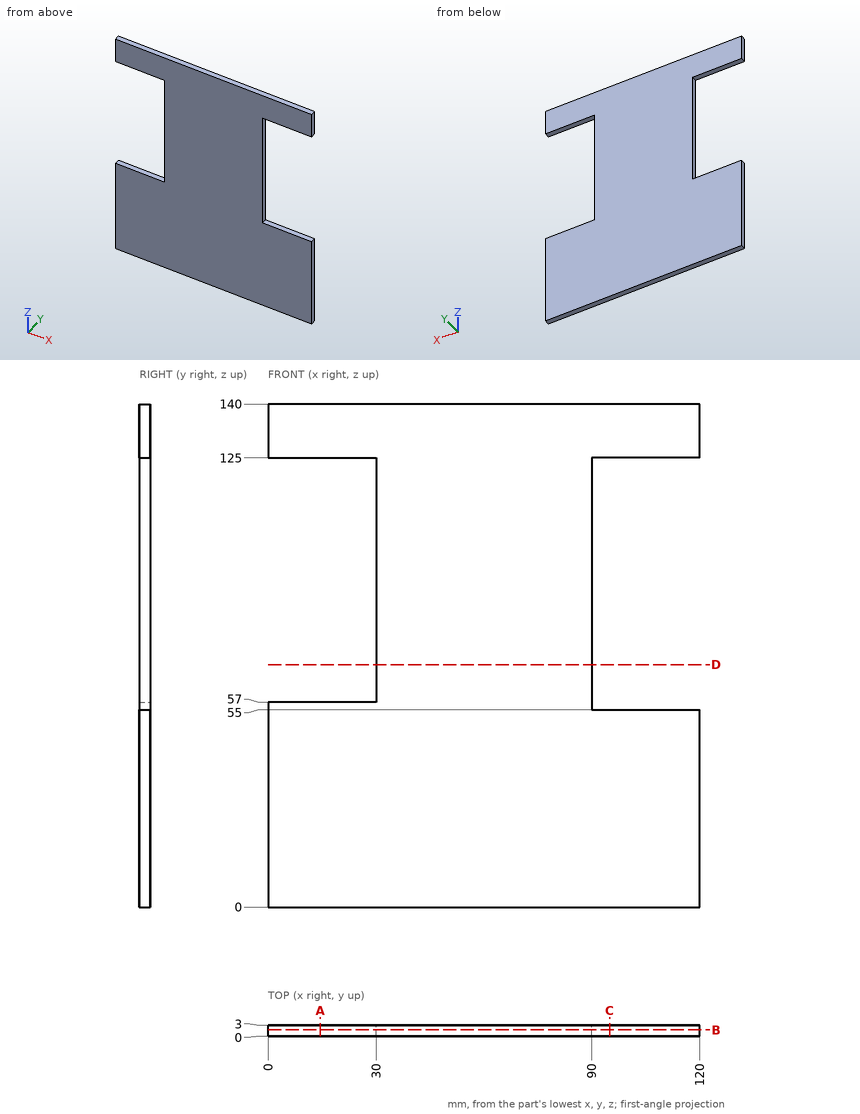
Source: three-view drawing plus pictorial views. Frame: mm from the lowest corner of the part. Coordinates: 2 decimals unless noted, no trailing zeros. Write each loop counter-clockwise with the first axis right and the second up, starting at its lowest first coordinate (ties: lowest second). Pieces come first, ordered by that corner, then holes. Notation, with made-up numbers: (62.5, 7) - (105.5, 7) arc R17 ccw to (105.5, 40) - close; hole circle Ø11 at (27.5, 58.5). An arc over 180 degrees is marked (long way). Answer as a JSON object with one key per item and string values.
Q1. Material intervals for line 1 (Z direction, x = 112.5, y = 1.85); line 2 (X direction, y = 2.85, z = 75.5), sorted ascending. Write a range as [from, to].
Ans:
{"line 1": "z = [0, 55], [125, 140]", "line 2": "x = [30, 90]"}
Q2. Section query A-A, the plane x = 14.5. Output: boundary loops of the cut face in (y, z), plus the area to 3 significant figures.
Ans:
{"outline": "(0, 0) - (3, 0) - (3, 57) - (0, 57) - close; (0, 125) - (3, 125) - (3, 140) - (0, 140) - close", "area": "216 mm2"}
Q3. Section query D-D, the plane z = 67.5. Output: boundary loops of the cut face in (x, y).
Ans:
{"outline": "(30, 0) - (90, 0) - (90, 3) - (30, 3) - close"}
Q4. Section query B-B, the plane y = 1.7. Output: boundary loops of the cut face in (x, z).
Ans:
{"outline": "(0, 0) - (120, 0) - (120, 55) - (90, 55) - (90, 125) - (120, 125) - (120, 140) - (0, 140) - (0, 125) - (30, 125) - (30, 57) - (0, 57) - close"}
Q5. Section query C-C, the plane x = 95. Output: boundary loops of the cut face in (y, z).
Ans:
{"outline": "(0, 0) - (3, 0) - (3, 55) - (0, 55) - close; (0, 125) - (3, 125) - (3, 140) - (0, 140) - close"}
